Design review of the part built by this model. Coordinates are the model's own, in mm. A direction names the side the tool comes from. Give positions to 0.01 mm unless a question says otherwise; leave off trailing zeros. Write each loop counter-clockwise with the first axis right and the second up, starting at its lowest first coordinate (ties: lowest second). Pieces come first, ordered by that corner, then holes. Notation, with made-up numbers: M 68,15 L 108,15 A35 cw 108,53 Z; hole C 58,-16 d10. An arc over 180 degrees is marked long. Answer in a Markdown table with one row per item.
```python
from build123d import *

# Parameters (mm, degrees)
SKETCH1_R           = 1.1
BOSS_EXTRUDE1_DEPTH = 2
BOSS_EXTRUDE3_START = -2
SKETCH3_R           = 3.75
SKETCH3_R_2         = 1.1
BOSS_EXTRUDE3_DEPTH = 2
CHAMFER1_SIZE       = 1.2
FILLET1_R           = 0.75


with BuildPart() as part:
    # Sketch1 → Boss-Extrude1 (new body)
    with BuildSketch(Plane(origin=(0, 0, 0), x_dir=(1, 0, 0), z_dir=(0, 1, 0))):
        with BuildLine():
            Line((-5, 3), (5, 3))
            ThreePointArc((5, 3), (8, 0), (5, -3))
            Line((5, -3), (-5, -3))
            ThreePointArc((-5, -3), (-8, 0), (-5, 3))
        make_face()
        with Locations(Location((-5, 0, 0), (0, 0, 270))):
            Circle(SKETCH1_R, mode=Mode.SUBTRACT)
        with Locations(Location((5, 0, 0), (0, 0, 270))):
            Circle(SKETCH1_R, mode=Mode.SUBTRACT)
    extrude(amount=BOSS_EXTRUDE1_DEPTH)

    # Sketch3 → Boss-Extrude3 (add)
    # profile 1 of 2: a face of its own
    with BuildSketch(Plane(origin=(0, 2, 0), x_dir=(1, 0, 0), z_dir=(0, 1, 0)).offset(BOSS_EXTRUDE3_START)):
        with Locations((-5, 0)):
            Circle(SKETCH3_R)
        with Locations(Location((-5, 0, 0), (0, 0, 270))):
            Circle(SKETCH3_R_2, mode=Mode.SUBTRACT)
    # profile 2 of 2: a face of its own
    with BuildSketch(Plane(origin=(0, 2, 0), x_dir=(1, 0, 0), z_dir=(0, 1, 0)).offset(BOSS_EXTRUDE3_START)):
        with Locations((5, 0)):
            Circle(SKETCH3_R)
        with Locations(Location((5, 0, 0), (0, 0, 270))):
            Circle(SKETCH3_R_2, mode=Mode.SUBTRACT)
    extrude(amount=BOSS_EXTRUDE3_DEPTH)

    # Chamfer1
    chamfer1_edges = [part.edges().sort_by_distance(p)[0] for p in [
        (-5, 2, -1.1),
        (5, 2, -1.1),
    ]]
    chamfer(chamfer1_edges, length=CHAMFER1_SIZE)

    # Fillet1
    fillet1_edges = [part.edges().sort_by_distance(p)[0] for p in [
        (0, 2, 3),
        (-8.75, 2, 0),
        (0, 2, -3),
        (8.75, 2, 0),
    ]]
    fillet(fillet1_edges, radius=FILLET1_R)


solid = part.part
```
1) Add section C-C (y = 0.4). Write out the cut boundary in (x, z), and give its area (3 significant figures).
Geometry says:
| item | result |
|---|---|
| outline | M -2.75,-3 L 2.75,-3 A3.75 ccw long 2.75,3 L -2.75,3 A3.75 ccw long Z; hole C -5,0 d2.2; hole C 5,0 d2.2 |
| area | 101 mm^2 |
2) For faces 4 (the face through (0, 1, -3)), 5 (the face through (0, 2, 0)), 6 (the face through (0, 1, 3)), list the 3-axis set-ups (+Z, -Z, +X, -X, +Y, -Y) from which the entire face can be reached by the end or side of a thin tool; tool diameter is ignored.
Geometry says:
| item | result |
|---|---|
| face 4 | -Z, +Y, -Y |
| face 5 | +Z, -Z, +X, -X, +Y |
| face 6 | +Z, +Y, -Y |
3) Add section D-D (x = 1). Write out the cut boundary in (y, z), and give its area (3 significant figures).
Geometry says:
| item | result |
|---|---|
| outline | M 0,-3 L 1.25,-3 A0.75 ccw 2,-2.25 L 2,2.25 A0.75 ccw 1.25,3 L 0,3 Z |
| area | 11.8 mm^2 |
4) Insertion check: P1, Ø1, axis at x = -1.5, z = -1, coming from the -Y side; P2, Ø0.6, axis at x = 1, y = 0.5, coming from the +Z side; P3, Ø0.6, axis at x = -1, y = 1, coming from the -Z side. Each pin has a flat end and moves straight along its axis. Give the tip position at first contact, or say it passes through.
Geometry says:
| item | result |
|---|---|
| P1 | y = 0 |
| P2 | z = 3 |
| P3 | z = -3 |
5) Add section A-A (z = 0). Write out the cut boundary in (x, y), and give its area (3 significant figures).
Geometry says:
| item | result |
|---|---|
| outline | M -8.75,0 L -6.1,0 L -6.1,0.8 L -7.3,2 L -8,2 A0.75 ccw -8.75,1.25 Z; M -3.9,0 L 3.9,0 L 3.9,0.8 L 2.7,2 L -2.7,2 L -3.9,0.8 Z; M 6.1,0 L 8.75,0 L 8.75,1.25 A0.75 ccw 8,2 L 7.3,2 L 6.1,0.8 Z |
| area | 23.1 mm^2 |
6) Add section B-B (x = -5). Write out the cut boundary in (y, z), and give its area (3 significant figures).
Geometry says:
| item | result |
|---|---|
| outline | M 0,-3.75 L 1.25,-3.75 A0.75 ccw 2,-3 L 2,-2.3 L 0.8,-1.1 L 0,-1.1 Z; M 0,1.1 L 0.8,1.1 L 2,2.3 L 2,3 A0.75 ccw 1.25,3.75 L 0,3.75 Z |
| area | 8.92 mm^2 |
7) To check wall thickness, follow probe 1 along X at (y, z) = (0.65, 0); probe 2 along X at (y, z) = (1.55, 1); probe 3 along X at (y, z) = (0.35, 2.25). State the ranges of each line that lie inside material, in increasing order. Write a range as [from, to].
Geometry says:
| item | result |
|---|---|
| probe 1 | [-8.75, -6.1], [-3.9, 3.9], [6.1, 8.75] |
| probe 2 | [-8.55, -6.56], [-3.44, 3.44], [6.56, 8.55] |
| probe 3 | [-8, 8] |
8) The part is to be moulded in two halves that separate along Z. For faces 1 (the face through (-3.91, 0.39, -0.14)), 2 (the face through (8.75, 0.62, 0.12)), 3 (the face through (0, 0, 0)), say which applies: released by +Z, released by -Z, zero draft, split by the parting line, or undercut.
Geometry says:
| item | result |
|---|---|
| face 1 | undercut |
| face 2 | split by the parting line |
| face 3 | zero draft |
